```python
from build123d import *

# Parameters (mm, degrees)
SKETCH2_R           = 45
SKETCH2_R_2         = 5
BOSS_EXTRUDE2_DEPTH = 25
CUT_EXTRUDE1_DEPTH  = 25


with BuildPart() as part:
    # Sketch2 → Boss-Extrude2 (new body)
    with BuildSketch(Plane.XY):
        with BuildLine():
            Line((107.0991595, 171.84228244), (-37.020034505, 40.675755006))
            ThreePointArc((-37.020034505, 40.675755006), (-54.235521991, -9.138279618), (-21.647362352, -50.560772375))
            Line((-21.647362352, -50.560772375), (109.894190801, -106.879683889))
            ThreePointArc((109.894190801, -106.879683889), (121.07607209, -104.578515845), (122.814256533, -93.295406417))
            Line((122.814256533, -93.295406417), (79.717724854, -5.126210099))
            ThreePointArc((79.717724854, -5.126210099), (78.265617309, 0.093033065), (78.780622712, 5.485980771))
            Line((78.780622712, 5.485980771), (123.44478962, 161.697643481))
            ThreePointArc((123.44478962, 161.697643481), (119.103356541, 172.943307617), (107.0991595, 171.84228244))
        make_face()
        Circle(SKETCH2_R, mode=Mode.SUBTRACT)
        with Locations((113.830074865, -97.686816185)):
            Circle(SKETCH2_R_2, mode=Mode.SUBTRACT)
        with Locations((113.830074865, 164.446690621)):
            Circle(SKETCH2_R_2, mode=Mode.SUBTRACT)
    extrude(amount=BOSS_EXTRUDE2_DEPTH)

    # Sketch3 → Cut-Extrude1 (cut)
    with BuildSketch(Plane.XY.offset(25)):
        with BuildLine():
            Line((17.795721205, 60.121434904), (62.437923836, 40.184140526))
            ThreePointArc((62.437923836, 40.184140526), (65.680023373, 40.175202237), (67.86378835, 42.571545249))
            Line((67.86378835, 42.571545249), (96.902891032, 129.688853296))
            ThreePointArc((96.902891032, 129.688853296), (95.288982132, 134.306972586), (90.41314241, 133.909587735))
            Line((90.41314241, 133.909587735), (16.731837096, 66.729574067))
            ThreePointArc((16.731837096, 66.729574067), (15.477705501, 63.137953736), (17.795721205, 60.121434904))
        make_face()
        with BuildLine():
            Line((27.085895713, -52.406577788), (62.496309368, -15.289638174))
            ThreePointArc((62.496309368, -15.289638174), (66.005561811, -14.098322429), (68.98684583, -16.2996928))
            Line((68.98684583, -16.2996928), (97.571155647, -75.006771443))
            ThreePointArc((97.571155647, -75.006771443), (96.977969452, -79.399977656), (92.696111536, -80.547942587))
            Line((92.696111536, -80.547942587), (28.701388064, -58.957803557))
            ThreePointArc((28.701388064, -58.957803557), (26.096410491, -56.125376983), (27.085895713, -52.406577788))
        make_face()
    extrude(amount=-CUT_EXTRUDE1_DEPTH, mode=Mode.SUBTRACT)


solid = part.part
```
Input: part model. Units: mm. Frame: model coordinates. A direction names the side the tool comes from. Give positions to 0.01 mm unless a question says otherwise; leave off trailing zeros. Order: outer loops, then holes, each group sorted by start corner. A loop starts at its lowest first (then second) coordinate and runs counter-clockwise, first axis right, second up. Notation, with made-up numbers: (-9.5, -6) - (0.5, -6) arc R17 cw to (0.5, 7) - close; hole circle Ø8 at (-29.75, 71). An arc over 180 degrees is marked (long way). One line per item, written item: value.
1. Cut plane B-B, the plane x = 59. Output: boundary loops of the cut face in (y, z), and give its area (3 significant figures).
Determined:
outline: (-85.09, 0) - (-69.18, 0) - (-69.18, 25) - (-85.09, 25) - close; (-18.95, 0) - (41.72, 0) - (41.72, 25) - (-18.95, 25) - close; (105.27, 0) - (128.07, 0) - (128.07, 25) - (105.27, 25) - close
area: 2,480 mm2
2. Draft query along X for faces 1 (the face through (20.765, -39.923, 12.325)), 2 (the face through (110.14, -94.31, 12.32)), 3 (the face through (54, 34, 0)), 4 (the face through (78.273, 0.017, 12.325)). Return one class per face: released by +X, released by -X, zero draft, split by the parting line, or undercut.
Determined:
face 1: undercut
face 2: undercut
face 3: zero draft
face 4: released by +X
3. Line query: probe 1 along Y at (x, z) = (28, 3); probe 2 along Y at (x, z) = (52, 2.5); probe 3 along X at (y, z) = (-34, 3). Output: solid intervals per line, ascending.
Determined:
probe 1: -71.82 to -58.64, -51.45 to -35.23, 35.23 to 55.56, 77 to 99.85
probe 2: -82.09 to -66.82, -26.29 to 44.85, 98.89 to 121.7
probe 3: -43.23 to -29.48, 29.48 to 44.65, 77.61 to 93.83
4. Cut plane A-A, the plane y = 0. Output: boundary loops of the cut face in (x, z).
Determined:
outline: (-55, 0) - (-45, 0) - (-45, 25) - (-55, 25) - close; (45, 0) - (78.27, 0) - (78.27, 25) - (45, 25) - close
5. Pin query (flat end, axial travel): pin 1 Ø5 at (y, z) = (77, 11.5) entering from +X; pin 2 Ø10 at (y, z) = (60, 6) entering from +X; pin 3 Ø1.5 at (x, z) = (9.5, 3) entering from +Y. Return the tip coordinate at first contact, or that it passes through.
Determined:
pin 1: x = 99.94
pin 2: x = 95.8
pin 3: y = 83.7
6. Cut plane C-C, the plane z = 9.5. Output: boundary loops of the cut face in (x, y), and give its area (3 significant figures).
Determined:
outline: (-37.02, 40.68) arc R55 ccw to (-21.65, -50.56) - (109.89, -106.88) arc R10 ccw to (122.81, -93.3) - (79.72, -5.13) arc R14.86 cw to (78.78, 5.49) - (123.44, 161.7) arc R10 ccw to (107.1, 171.84) - close; hole circle Ø90 at (0, 0); hole (16.73, 66.73) arc R4 ccw to (17.8, 60.12) - (62.44, 40.18) arc R4 ccw to (67.86, 42.57) - (96.9, 129.69) arc R4 ccw to (90.41, 133.91) - close; hole (27.09, -52.41) arc R4 ccw to (28.7, -58.96) - (92.7, -80.55) arc R4 ccw to (97.57, -75.01) - (68.99, -16.3) arc R4 ccw to (62.5, -15.29) - close; hole circle Ø10 at (113.83, -97.69); hole circle Ø10 at (113.83, 164.45)
area: 13,600 mm2
7. Cut plane D-D, the plane x = 0. Output: boundary loops of the cut face in (y, z), and give its area (3 significant figures).
Determined:
outline: (-59.83, 0) - (-45, 0) - (-45, 25) - (-59.83, 25) - close; (45, 0) - (74.37, 0) - (74.37, 25) - (45, 25) - close
area: 1,100 mm2
8. Reachability of faces 5 (the face through (100.8, 82.5, 12.3)), 6 (the face through (82.18, 85.52, 12.68)), 7 (the face through (-54.358, -8.379, 12.325)) from +Z, -Z, +X, -X, +Y, -Y: full face, straight path, thin tool, end or side. Return the list, or none.
Determined:
face 5: +Z, -Z, +X
face 6: +Z, -Z
face 7: +Z, -Z, -X
